```python
from build123d import *

# Parameters (mm, degrees)
SKETCH_1_R                       = 1.15
EXTRUDE_1_DEPTH                  = 4
FILLET_1_R                       = 2
REVOLVE_START                    = -30
REVOLVE_2_DEPTH                  = 20
PATTERN_CIRCULAR_4_COUNT         = 2
PATTERN_CIRCULAR_4_ANGLE         = 83
FILLET_1_OF_PATTERN_CIRCULAR_4_R = 2
FILLET_2_R                       = 1
FILLET_3_R                       = 2


# Read off the part's stored shape, not the designer's step: the revolve step
with BuildPart() as part:
    # Sketch 1 → Extrude 1 (new body)
    # profile 1 of 2: a face of its own
    with BuildSketch(Plane(origin=(0, 0, 0), x_dir=(1, 0, 0), z_dir=(0, 1, 0))):
        Polygon((25, 40), (25, 30), (25, 20.100505063), (30.563454525, 25.663959588), (30.563454525, 37.663959588), (36, 43.100505063), (36, 65), (30, 65), (30, 45), align=None)
        with Locations(Location((33, 52, 0), (0, 0, 270))):
            Circle(SKETCH_1_R, mode=Mode.SUBTRACT)
        with Locations(Location((33, 60, 0), (0, 0, 270))):
            Circle(SKETCH_1_R, mode=Mode.SUBTRACT)
    # profile 2 of 2: a face of its own
    with BuildSketch(Plane(origin=(0, 0, 0), x_dir=(1, 0, 0), z_dir=(0, 1, 0))):
        Polygon((30.563454525, 25.663959588), (25, 20.100505063), (25, 10), (30.563454525, 10), align=None)
    extrude_1 = extrude(amount=EXTRUDE_1_DEPTH)

    # Fillet 1
    fillet_1_edges = [part.edges().sort_by_distance(p)[0] for p in [
        (30, 2, -45),
        (30, 2, -65),
        (36, 2, -65),
        (36, 2, -43.100505063),
        (30.563454525, 2, -37.663959588),
    ]]
    fillet(fillet_1_edges, radius=FILLET_1_R)

    # Revolve 2 outline → Revolve 2 (add)
    with BuildSketch(Plane.XY.offset(REVOLVE_START)):
        with BuildLine():
            Line((-12.431276894, 29.921105051), (-10.168416077, 24.838636441))
            ThreePointArc((-10.168416077, 24.838636441), (13.615975876, 22.966764198), (25, 1.999999999))
            Line((25, 1.999999999), (25, 4))
            Line((25, 4), (30.497946693, 4))
            ThreePointArc((30.497946693, 4), (15.79800814, 28.163862317), (-12.431276894, 29.921105051))
        make_face()
        with BuildLine():
            Line((25, 0), (25, 1.999999999))
            ThreePointArc((25, 1.999999999), (24.09076133, -4.680959403), (21.429182518, -10.875951873))
            Line((21.429182518, -10.875951873), (26.197993815, -13.741342781))
            ThreePointArc((26.197993815, -13.741342781), (29.168708283, -7.127497445), (30.497946693, 0))
            Line((30.497946693, 0), (25, 0))
        make_face()
    extrude(amount=REVOLVE_2_DEPTH)

    # Pattern Circular 4: Extrude 1 ×2 about axis
    pattern_circular_4_axis = Axis((0, 2, 0), (0, 0, 1))
    for i in range(1, PATTERN_CIRCULAR_4_COUNT):
        add(extrude_1.rotate(pattern_circular_4_axis, i * PATTERN_CIRCULAR_4_ANGLE / (PATTERN_CIRCULAR_4_COUNT - 1)))

    # Fillet 1 of Pattern Circular 4
    fillet_1_of_pattern_circular_4_edges = [part.edges().sort_by_distance(p)[0] for p in [
        (3.656080302, 31.776384549, -45),
        (3.656080302, 31.776384549, -65),
        (4.387296363, 37.731661459, -65),
        (4.387296363, 37.731661459, -43.100505063),
        (3.724748135, 32.335639169, -37.663959588),
    ]]
    fillet(fillet_1_of_pattern_circular_4_edges, radius=FILLET_1_OF_PATTERN_CIRCULAR_4_R)

    # Fillet 2
    fillet_2_edges = [part.edges().sort_by_distance(p)[0] for p in [
        (13.615975876, 22.966764198, -10),
        (29.168708283, -7.127497445, -10),
        (-5.504691137, 32.063651275, -10),
        (22.890674114, 22.251957711, -10),
    ]]
    fillet(fillet_2_edges, radius=FILLET_2_R)

    # Fillet 3
    fillet_3_edges = [part.edges().sort_by_distance(p)[0] for p in [
        (5.366841465, 29.298398021, -30),
        (1.396656859, 29.785875394, -30),
        (27.748973347, 0, -30),
        (27.748973347, 4, -30),
    ]]
    fillet(fillet_3_edges, radius=FILLET_3_R)


solid = part.part
```
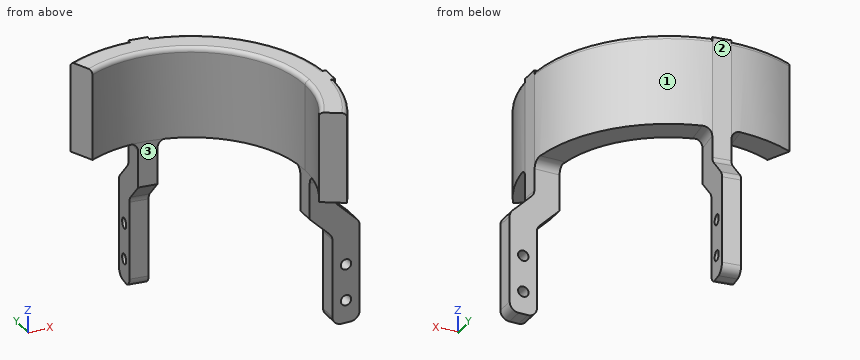
Geometry: final body of the model. Coordinates: model frame, mm. Face numbers are marked on the shaded views. A direction names the side the tool comes from. Coordinates: 2 decimals unless noted, no trailing zeros. Order: outer loops, then holes, each group sorted by start corner. A loop starts at its lowest first (then second) coordinate and runs counter-clockwise, first axis right, second up. Notation, with made-up numbers: M 24.5,-4.5 L 46.5,-4.5 A5 cw 46.5,3.5 Z; hole C 80.5,49 d9. An arc over 180 degrees is marked long. Answer as CSV lines item,"result".
Q1. Section C-C on z = -15. Return the cut outline in (x, y).
Answers:
outline,"M -12.43,29.92 L -10.17,24.84 A25 cw 21.43,-10.88 L 26.2,-13.74 A30.56 ccw 30.5,0 L 30.56,0 L 30.56,4 L 30.5,4 A30.56 ccw 5.7,32.03 L 5.71,32.09 L 1.74,32.58 L 1.73,32.51 A30.56 ccw Z"
Q2. Line query: probe 1 along X at (y, z) = (1.95, -60); probe 2 along Y at (x, z) = (30.5, -41); probe 3 along X at (y, z) = (2.5, -18.5) (3 decimals). Output: solid intervals per line, ascending. Write a range as [from, to].
Answers:
probe 1,"x = [30, 31.85], [34.15, 36]"
probe 2,"y = [0, 4]"
probe 3,"x = [24.995, 30.563]"
Q3. Section B-B on z = -60. Return the cut outline in (x, y).
Answers:
outline,"M 1.67,32.02 L 5.64,31.53 L 5.87,33.37 L 1.9,33.86 Z; M 2.18,36.14 L 6.15,35.65 L 6.37,37.49 L 2.4,37.98 Z; M 30,0 L 31.85,0 L 31.85,4 L 30,4 Z; M 34.15,0 L 36,0 L 36,4 L 34.15,4 Z"
Q4. Section A-A on x = 33. Return the cut outline in (y, z).
Answers:
outline,"M 0,-65 L 4,-65 L 4,-61.15 L 0,-61.15 Z; M 0,-58.85 L 4,-58.85 L 4,-53.15 L 0,-53.15 Z; M 0,-50.85 L 4,-50.85 L 4,-40.1 L 0,-40.1 Z"
Q5. Set-up query: the marked faces 1, 2 and 3. Return all of +Z, -Z, +X, -X, +Y, -Y with unobstructed straight access to the full face (end or side cutting, diameter ignored); none if empty.
Answers:
face 1,"+Z, -Z, +X, +Y"
face 2,"+Z, +X, +Y"
face 3,"-Z, -X, -Y"
Q6. First-contact query: P1, Ø4.5, axis at x = 27.5, y = -5.5, coming from the -Z side; P2, Ø4, axis at y = 28, z = -37, coming from the -X side; P3, Ø4.5, axis at y = 2, z = -51.5, coming from the -X side. Flat tips, straight axial feed; report the tip coordinate or a pass-through.
Answers:
P1,"stops at z = -30"
P2,"stops at x = 1.06"
P3,"stops at x = 30"
